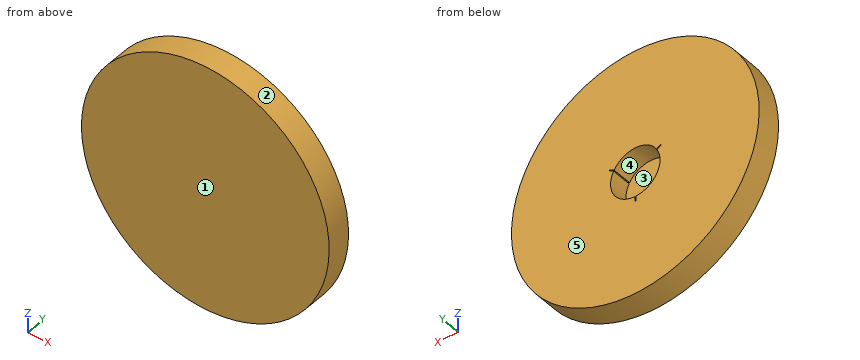
```python
from build123d import *

# Parameters (mm, degrees)
SKETCH_2_R      = 125
EXTRUDE_1_DEPTH = 25
SKETCH_3_R      = 125
EXTRUDE_2_DEPTH = 5


with BuildPart() as part:
    # 草圖2 → 填料-伸長1 (new body)
    with BuildSketch(Plane(origin=(0, 0, 0), x_dir=(1, 0, 0), z_dir=(0, 1, 0))):
        with Locations(Location((0, 0, 0), (0, 0, 270))):
            Circle(SKETCH_2_R)
        with BuildLine():
            Line((26.226431553, -14.564487048), (25.726431553, -15.430512452))
            Line((25.726431553, -15.430512452), (21.396304534, -12.930512452))
            ThreePointArc((21.396304534, -12.930512452), (0, -25), (-21.396304534, -12.930512452))
            Line((-21.396304534, -12.930512452), (-25.726431553, -15.430512452))
            Line((-25.726431553, -15.430512452), (-26.226431553, -14.564487048))
            Line((-26.226431553, -14.564487048), (-21.896304534, -12.064487048))
            ThreePointArc((-21.896304534, -12.064487048), (-21.650635095, 12.5), (-0.5, 24.9949995))
            Line((-0.5, 24.9949995), (-0.5, 29.9949995))
            Line((-0.5, 29.9949995), (0.5, 29.9949995))
            Line((0.5, 29.9949995), (0.5, 24.9949995))
            ThreePointArc((0.5, 24.9949995), (21.650635095, 12.5), (21.896304534, -12.064487048))
            Line((21.896304534, -12.064487048), (26.226431553, -14.564487048))
        make_face(mode=Mode.SUBTRACT)
    extrude(amount=EXTRUDE_1_DEPTH)

    # 草圖3 → 填料-伸長2 (add)
    with BuildSketch(Plane.XZ):
        with Locations(Location((0, 0, 0), (0, 0, 90))):
            Circle(SKETCH_3_R)
    extrude(amount=-EXTRUDE_2_DEPTH)


solid = part.part
```
CAD build for the part. Positions are in the model's coordinates, mm. Face numbers are marked on the shaded views. A direction names the side the tool comes from. Coordinates: 2 decimals unless noted, no trailing zeros. Loops run counter-clockwise (first coordinate to the right, second up) from the corner with the lowest first, then second, coordinate; pieces in that order, holes last. Notation, with made-up numbers: (74, -1) - (103, -1) arc R19 cw to (103, 3) - close; hole circle Ø1 at (35.25, 41). An arc over 180 degrees is marked (long way). Return JSON: item names as keys, results as strings.
1. Band-saw the part on B-B (y = 10.25). Give the cut face in (x, z) (3 decimals).
Result:
{"outline": "circle Ø250 at (0, 0); hole (-26.226, 14.564) - (-21.896, 12.064) arc R25 ccw to (-0.5, -24.995) - (-0.5, -29.995) - (0.5, -29.995) - (0.5, -24.995) arc R25 ccw to (21.896, 12.064) - (26.226, 14.564) - (25.726, 15.431) - (21.396, 12.931) arc R25 ccw to (-21.396, 12.931) - (-25.726, 15.431) - close"}
2. Band-saw the part on D-D (z = 75). Give the cut face in (x, y).
Result:
{"outline": "(-100, 0) - (100, 0) - (100, 25) - (-100, 25) - close"}
3. Drop flat-ended pins along their axis: pin 1 (1 mm diameter, centred on x = 41, z = -76.5, fed in from -Y); pin 2 (15.5 mm diameter, centred on x = -0.5, z = -3, fed in from +Y); pin 3 (5.5 mm diameter, centred on y = 17, z = -27, fed in from -X); pin 4 (3 mm diameter, centred on x = 28, y = 22.5, fed in from +Z). Give the stop position or say it passes through.
Result:
{"pin 1": "stops at y = 0", "pin 2": "stops at y = 5", "pin 3": "stops at x = -122.63", "pin 4": "stops at z = 122.16"}
4. Band-saw the part on C-C (x = 12.5). Give the cut face in (y, z).
Result:
{"outline": "(0, -124.37) - (25, -124.37) - (25, -21.65) - (5, -21.65) - (5, 21.65) - (25, 21.65) - (25, 124.37) - (0, 124.37) - close"}
5. 3-axis set-ups, long thin cutter, end or side, ignore diameter. For the marked faces 4 and 5: which of +Z, -Z, +X, -X, +Y, -Y reach the whole face in a straight line?
Result:
{"face 4": "+Y", "face 5": "+Z, -Z, +X, -X, +Y"}
6. Probe L1, parallel to Z at x = 22, y = 18.75; L2, parallel to Z at x = -12, y = 11.75; L3, parallel to X at y = 19.25, z = 6. List the from-to ranges inside material, lowest first. Write a range as from..to.
Result:
{"L1": "z = -123.05..-11.87, 11.87..12.12, 13.28..123.05", "L2": "z = -124.42..-21.93, 21.93..124.42", "L3": "x = -124.86..-24.27, 24.27..124.86"}
7. Band-saw the part on A-A (z = 0). Give the cut face in (x, y).
Result:
{"outline": "(-125, 0) - (125, 0) - (125, 25) - (25, 25) - (25, 5) - (-25, 5) - (-25, 25) - (-125, 25) - close"}
8. Mould opens along Y. For the marked faces 1, 2 and 3 say: released by +Y, released by -Y, zero draft, split by the parting line, or undercut.
Result:
{"face 1": "released by -Y", "face 2": "zero draft", "face 3": "released by +Y"}
